Geometry: final body of the model. Coordinates: model frame, mm. Face numbers are marked on the shaded views. A direction names the side the tool comes from. Give positions to 0.01 mm unless a question says otherwise; leave off trailing zeros. Loops run counter-clockwise (first coordinate to the right, second up) from the corner with the lowest first, then second, coordinate; pieces in that order, holes last. Notation, with made-up numbers: (19, 64.25) - (72, 64.25) arc R21 ccw to (72, 99.25) - close; hole circle Ø1 at (41.25, 70.25). An arc over 180 degrees is marked (long way). Use one line per item in the form item = value.
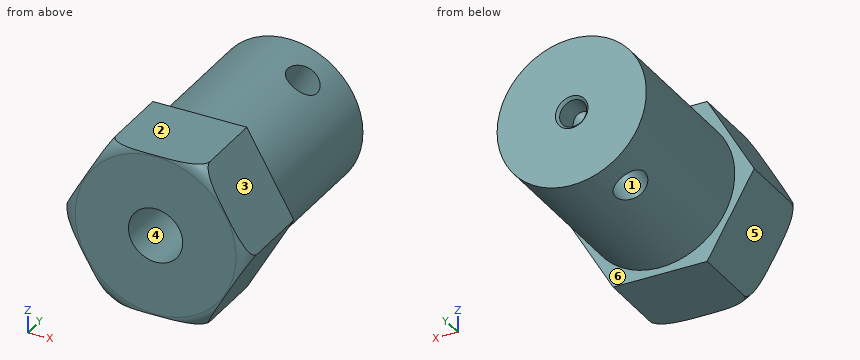
```python
from build123d import *

# Parameters (mm, degrees)
SKETCH1_R                = 2
BASE_DEPTH               = 6
SKETCH2_R                = 5.5
SHAFT_HOLDING_BODY_DEPTH = 12
M3X0_5_1_D               = 2.5
SKETCH13_R               = 1
SHAFT_HOLE_DEPTH         = 19.0000001
SH_C_SIZE                = 0.2


with BuildPart() as part:
    # Sketch1 → BASE (new body)
    with BuildSketch(Plane(origin=(0, 0, 0), x_dir=(1, 0, 0), z_dir=(0, 1, 0))):
        Polygon((3.464101615, -6), (6.92820323, 0), (3.464101615, 6), (-3.464101615, 6), (-6.92820323, 0), (-3.464101615, -6), align=None)
        Circle(SKETCH1_R, mode=Mode.SUBTRACT)
    extrude(amount=BASE_DEPTH)

    # Sketch2 → SHAFT HOLDING BODY (add)
    with BuildSketch(Plane(origin=(0, 6, 0), x_dir=(1, 0, 0), z_dir=(0, 1, 0))):
        Circle(SKETCH2_R)
    extrude(amount=SHAFT_HOLDING_BODY_DEPTH)

    # M3x0.5 螺纹孔1 (through all)
    with Locations(Plane(origin=(2.75, 6, 4.763139721), x_dir=(0.866025404, 0, -0.5), z_dir=(0.5, 0, 0.866025404))):
        with Locations((0, 9)):
            Hole(M3X0_5_1_D / 2)

    # Sketch9 → BASE CHAMFER RELIEF (revolve, cut)
    with BuildSketch(Plane.XY):
        with BuildLine():
            Line((-6.92820323, 1), (-6.92820323, 0))
            Line((-6.92820323, 0), (-5.92820323, 0))
            ThreePointArc((-5.92820323, 0), (-6.635310011, 0.292893219), (-6.92820323, 1))
        make_face()
    revolve(axis=Axis((0, 22.106901259, 0), (0, -1, 0)), mode=Mode.SUBTRACT)

    # Sketch13 → SHAFT HOLE (cut, through all)
    with BuildSketch(Plane(origin=(0, 18, 0), x_dir=(1, 0, 0), z_dir=(0, 1, 0))):
        Circle(SKETCH13_R)
    extrude(amount=-SHAFT_HOLE_DEPTH, mode=Mode.SUBTRACT)

    # SH C
    sh_c_edges = [part.edges().sort_by_distance(p)[0] for p in [
        (-1, 18, 0),
    ]]
    chamfer(sh_c_edges, length=SH_C_SIZE)


solid = part.part
```
(1) Cut plane B-B (y = 8.5). Return the cut outline in (x, z), plus the area to 3 significant figures.
Solution:
outline = circle Ø11 at (0, 0); hole circle Ø2 at (0, 0)
area = 91.9 mm2
(2) Access query for the marked faces 5 and 6. Directions: +Z, -Z, +X, -X, +Y, -Y. A direction counts if a zero-diameter tool reaches every point of the face in a straight line with its end or side. Return the directions, or none.
Solution:
face_5 = -Z, -X, +Y, -Y
face_6 = +Y
(3) Pull-direction query (X, two-part tool) for the marked faces 1, 2, 3 and 4; classes: released by +X, released by -X, zero draft, split by the parting line, or undercut.
Solution:
face_1 = undercut
face_2 = zero draft
face_3 = released by +X
face_4 = undercut
(4) Cut plane A-A (y = 4). Return the cut outline in (x, z), plus the area to 3 significant figures.
Solution:
outline = (-6.93, 0) - (-3.46, -6) - (3.46, -6) - (6.93, 0) - (3.46, 6) - (-3.46, 6) - close; hole circle Ø4 at (0, 0)
area = 112 mm2
(5) Material intervals for L1, parallel to X at y = 16.35, z = 0; L2, parallel to Z at x = 0, y = 3.45, sorted ascending. Write a range as from..to.
Solution:
L1 = -5.5..-1, 1..5.5
L2 = -6..-2, 2..6
(6) Pin query (flat end, axial travel): P1, Ø1.5, axis at x = -3, y = 12, coming from the -Z side; P2, Ø3, axis at x = 0, z = 0, coming from the -Y side; P3, Ø2, axis at x = -2.5, y = 11, coming from the -Z side. Return the tip coordinate at first contact, or that it passes through.
Solution:
P1 = -5.02
P2 = 6
P3 = -5.29
